```python
from build123d import *

# Parameters (mm, degrees)
SKETCH_1_W          = 178
SKETCH_1_H          = 42.5
SKETCH_1_R          = 2.1
EXTRUDE_1_DEPTH     = 3
FILLET_1_R          = 3
CUT_EXTRUDE_1_DEPTH = 10


with BuildPart() as part:
    # 草图1 → 凸台-拉伸1 (new body)
    with BuildSketch(Plane.XY):
        with Locations((0, 5.001204258)):
            Rectangle(SKETCH_1_W, SKETCH_1_H)
        with Locations((-83, 15.751204258)):
            Circle(SKETCH_1_R, mode=Mode.SUBTRACT)
        with Locations((-83, -4.248795742)):
            Circle(SKETCH_1_R, mode=Mode.SUBTRACT)
        with Locations((-47.5, 11.751204258)):
            Circle(SKETCH_1_R, mode=Mode.SUBTRACT)
        with Locations((47.5, 11.751204258)):
            Circle(SKETCH_1_R, mode=Mode.SUBTRACT)
        with Locations((47.5, -13.248795742)):
            Circle(SKETCH_1_R, mode=Mode.SUBTRACT)
        with Locations((-47.5, -13.248795742)):
            Circle(SKETCH_1_R, mode=Mode.SUBTRACT)
        with Locations(Location((83, -4.248795742, 0), (0, 0, 180))):
            Circle(SKETCH_1_R, mode=Mode.SUBTRACT)
        with Locations(Location((83, 15.751204258, 0), (0, 0, 180))):
            Circle(SKETCH_1_R, mode=Mode.SUBTRACT)
    extrude(amount=EXTRUDE_1_DEPTH)

    # 圆角1
    fillet_1_edges = [part.edges().sort_by_distance(p)[0] for p in [
        (-89, 26.251204258, 1.5),
        (89, 26.251204258, 1.5),
        (89, -16.248795742, 1.5),
        (-89, -16.248795742, 1.5),
    ]]
    fillet(fillet_1_edges, radius=FILLET_1_R)

    # 草图2 → 切除-拉伸1 (cut)
    with BuildSketch(Plane.XY.offset(3)):
        with BuildLine():
            Line((-73, 19.001204258), (-73, -8.998795742))
            ThreePointArc((-73, -8.998795742), (-75, -10.998795742), (-77, -8.998795742))
            Line((-77, -8.998795742), (-77, 19.001204258))
            ThreePointArc((-77, 19.001204258), (-75, 21.001204258), (-73, 19.001204258))
        make_face()
        with BuildLine():
            Line((-67, 19.001204258), (-67, -8.998795742))
            ThreePointArc((-67, -8.998795742), (-65, -10.998795742), (-63, -8.998795742))
            Line((-63, -8.998795742), (-63, 19.001204258))
            ThreePointArc((-63, 19.001204258), (-65, 21.001204258), (-67, 19.001204258))
        make_face()
        with BuildLine():
            Line((-57, 19.001204258), (-57, -8.998795742))
            ThreePointArc((-57, -8.998795742), (-55, -10.998795742), (-53, -8.998795742))
            Line((-53, -8.998795742), (-53, 19.001204258))
            ThreePointArc((-53, 19.001204258), (-55, 21.001204258), (-57, 19.001204258))
        make_face()
        with BuildLine():
            Line((-37, 19.001204258), (-37, -8.998795742))
            ThreePointArc((-37, -8.998795742), (-35, -10.998795742), (-33, -8.998795742))
            Line((-33, -8.998795742), (-33, 19.001204258))
            ThreePointArc((-33, 19.001204258), (-35, 21.001204258), (-37, 19.001204258))
        make_face()
        with BuildLine():
            Line((-27, 19.001204258), (-27, -8.998795742))
            ThreePointArc((-27, -8.998795742), (-25, -10.998795742), (-23, -8.998795742))
            Line((-23, -8.998795742), (-23, 19.001204258))
            ThreePointArc((-23, 19.001204258), (-25, 21.001204258), (-27, 19.001204258))
        make_face()
        with BuildLine():
            Line((-17, 19.001204258), (-17, -8.998795742))
            ThreePointArc((-17, -8.998795742), (-15, -10.998795742), (-13, -8.998795742))
            Line((-13, -8.998795742), (-13, 19.001204258))
            ThreePointArc((-13, 19.001204258), (-15, 21.001204258), (-17, 19.001204258))
        make_face()
        with BuildLine():
            Line((-7, 19.001204258), (-7, -8.998795742))
            ThreePointArc((-7, -8.998795742), (-5, -10.998795742), (-3, -8.998795742))
            Line((-3, -8.998795742), (-3, 19.001204258))
            ThreePointArc((-3, 19.001204258), (-5, 21.001204258), (-7, 19.001204258))
        make_face()
        with BuildLine():
            Line((3, 19.001204258), (3, -8.998795742))
            ThreePointArc((3, -8.998795742), (5, -10.998795742), (7, -8.998795742))
            Line((7, -8.998795742), (7, 19.001204258))
            ThreePointArc((7, 19.001204258), (5, 21.001204258), (3, 19.001204258))
        make_face()
        with BuildLine():
            Line((13, 19.001204258), (13, -8.998795742))
            ThreePointArc((13, -8.998795742), (15, -10.998795742), (17, -8.998795742))
            Line((17, -8.998795742), (17, 19.001204258))
            ThreePointArc((17, 19.001204258), (15, 21.001204258), (13, 19.001204258))
        make_face()
        with BuildLine():
            Line((23, 19.001204258), (23, -8.998795742))
            ThreePointArc((23, -8.998795742), (25, -10.998795742), (27, -8.998795742))
            Line((27, -8.998795742), (27, 19.001204258))
            ThreePointArc((27, 19.001204258), (25, 21.001204258), (23, 19.001204258))
        make_face()
        with BuildLine():
            Line((33, 19.001204258), (33, -8.998795742))
            ThreePointArc((33, -8.998795742), (35, -10.998795742), (37, -8.998795742))
            Line((37, -8.998795742), (37, 19.001204258))
            ThreePointArc((37, 19.001204258), (35, 21.001204258), (33, 19.001204258))
        make_face()
        with BuildLine():
            Line((53, 19.001204258), (53, -8.998795742))
            ThreePointArc((53, -8.998795742), (55, -10.998795742), (57, -8.998795742))
            Line((57, -8.998795742), (57, 19.001204258))
            ThreePointArc((57, 19.001204258), (55, 21.001204258), (53, 19.001204258))
        make_face()
        with BuildLine():
            Line((63, 19.001204258), (63, -8.998795742))
            ThreePointArc((63, -8.998795742), (65, -10.998795742), (67, -8.998795742))
            Line((67, -8.998795742), (67, 19.001204258))
            ThreePointArc((67, 19.001204258), (65, 21.001204258), (63, 19.001204258))
        make_face()
        with BuildLine():
            Line((73, 19.001204258), (73, -8.998795742))
            ThreePointArc((73, -8.998795742), (75, -10.998795742), (77, -8.998795742))
            Line((77, -8.998795742), (77, 19.001204258))
            ThreePointArc((77, 19.001204258), (75, 21.001204258), (73, 19.001204258))
        make_face()
    extrude(amount=-CUT_EXTRUDE_1_DEPTH, mode=Mode.SUBTRACT)


solid = part.part
```
Could you check a few things on this model? Use its own coordinates, in mm. A direction names the side the tool comes from. Coordinates: 2 decimals unless noted, no trailing zeros. Order: outer loops, then holes, each group sorted by start corner. A loop starts at its lowest first (then second) coordinate and runs counter-clockwise, first axis right, second up. Notation, with made-up numbers: M -38,33 L 10,33 A27 ccw 10,62 Z; hole C 13.5,59.25 d4. An arc over 180 degrees is marked long. Use one line per item in the form item = value. Start each with the question number.
1. Suppose I cut it at A-A on x = -83. Write out the boundary of the cut face in (y, z).
2. Suppose I cut it at B-B on x = 55. Write out the boundary of the cut face in (y, z).
3. We'd pull the mould along Y, two halves only. Please class faces 3 (the flat face through (89, 5, 1)), 4 (the flat face through (-1, -16.249, 1)), 5 (the flat face through (73, 5, 2)): +Y half, -Y half, draft (parallel to the pull), parting line (faces both ways), or undercut.
4. Suppose I cut it at C-C on z = 2.35. Count the separate pieces of the cut face and the enclosed holes in it, then the cut area to 3 significant figures.
5. On a 3-axis mill with a long thin cutter (end or side, diameter ignored), from which of +Z, -Z, +X, -X, +Y, -Y can I reach the whole of each face in a straight line? I mean faces 1 (the cylindrical face through (88.098, 25.396, 1.521)), 2 (the flat face through (53, 5, 2)). Say none if no direction works.
6. Please list where these lines run through material, in increasing order: line 1 (Y direction, x = 83, z = 1.35); line 2 (Y direction, x = -47.5, z = 2.1); line 3 (X direction, y = -11.5, z = 2.4).
7. For pin 1 (4 mm diameter, centred on x = -47.5, y = 11.75, fed in from -Z), with a flat end and sliding along its axis, tell me the tip position at first contact or that it passes through.
Geometry says:
q1.outline = M -16.25,0 L -6.35,0 L -6.35,3 L -16.25,3 Z; M -2.15,0 L 13.65,0 L 13.65,3 L -2.15,3 Z; M 17.85,0 L 26.25,0 L 26.25,3 L 17.85,3 Z
q2.outline = M -16.25,0 L -11,0 L -11,3 L -16.25,3 Z; M 21,0 L 26.25,0 L 26.25,3 L 21,3 Z
q3.face_3 = draft
q3.face_4 = -Y half
q3.face_5 = undercut
q4.separate_pieces = 1
q4.enclosed_holes = 22
q4.area = 5,700 mm^2
q5.face_1 = +Z, -Z, +X, +Y
q5.face_2 = +Z, -Z
q6.line_1 = -16.25 to -6.35, -2.15 to 13.65, 17.85 to 26.25
q6.line_2 = -16.25 to -15.35, -11.15 to 9.65, 13.85 to 26.25
q6.line_3 = -89 to -48.66, -46.34 to 46.34, 48.66 to 89
q7.pin_1 = through
